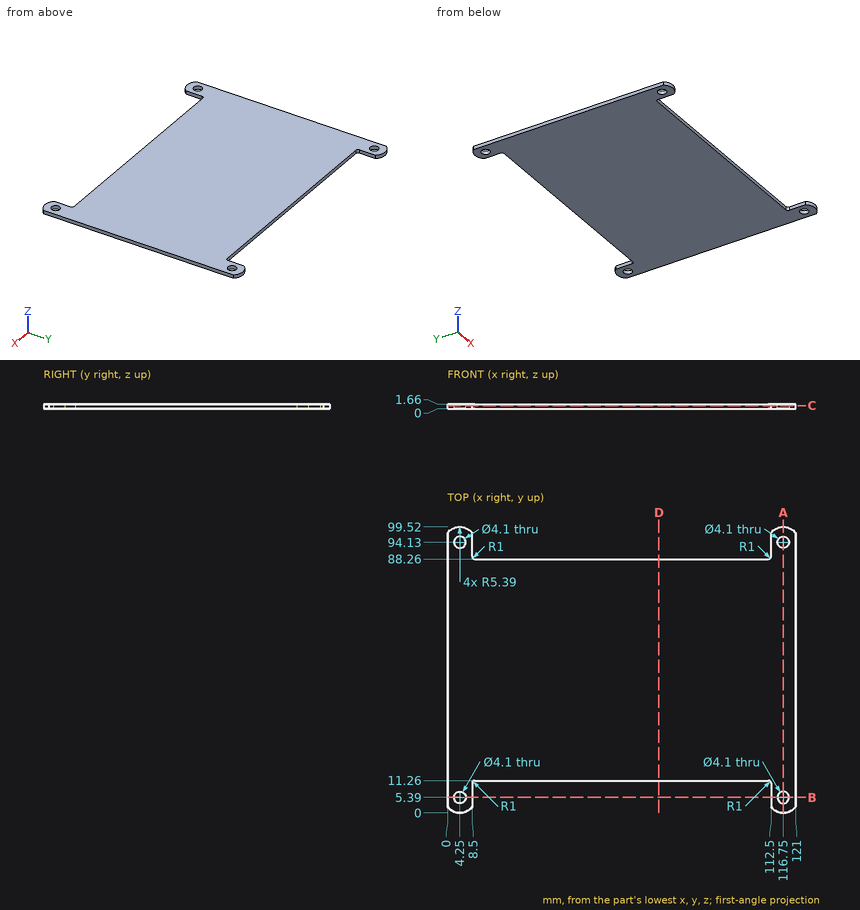
Verification items for this drawing (mm, ordinates from the low corner). Coordinates: 2 decimals unless noted, no trailing zeros. Write each loop counter-clockwise with the first axis right and the second up, starting at its lowest first coordinate (ties: lowest second). Pieces come first, ordered by that corner, then holes. Notation, with made-up numbers: (-18, 20.5) -> (8, 20.5) arc R26 cw to (8, 51.5) -> close; hole circle Ø11 at (78.5, 24.5). An arc over 180 degrees is marked (long way). One line per item, written item: value. Start each with the question number.
Q1. Cross-section at C-C on z = 1.1. Enter the section's corners in (x, y).
Q2. Thickness scan on L1, parallel to X at y = 94.13, z = 0.6; L2, parallel to X at y = 93.5, z = 0.35; L3, parallel to Y at x = 34.5, z = 0.4. Record the ranges inside material, lowest first. Write a range as from..to.
Q3. Cross-section at D-D on x = 73.5. Enter the section's corners in (y, z).
Q4. Cross-section at A-A on x = 116.75. Enter the section's corners in (y, z).
Q5. Cross-section at B-B on y = 5.39. Enter the section's corners in (x, z), and give its area (3 significant figures).
Checked values:
1. outline: (0, 2.07) arc R5.39 ccw to (8.5, 2.07) -> (8.5, 10.26) arc R1 cw to (9.5, 11.26) -> (111.5, 11.26) arc R1 cw to (112.5, 10.26) -> (112.5, 2.07) arc R5.39 ccw to (121, 2.07) -> (121, 97.45) arc R5.39 ccw to (112.5, 97.45) -> (112.5, 89.26) arc R1 cw to (111.5, 88.26) -> (9.5, 88.26) arc R1 cw to (8.5, 89.26) -> (8.5, 97.45) arc R5.39 ccw to (0, 97.45) -> close; hole circle Ø4.1 at (4.25, 5.39); hole circle Ø4.1 at (4.25, 94.13); hole circle Ø4.1 at (116.75, 5.39); hole circle Ø4.1 at (116.75, 94.13)
2. L1: x = 0..2.2, 6.3..8.5, 112.5..114.7, 118.8..121
2. L2: x = 0..2.3, 6.2..8.5, 112.5..114.8, 118.7..121
2. L3: y = 11.26..88.26
3. outline: (11.26, 0) -> (88.26, 0) -> (88.26, 1.66) -> (11.26, 1.66) -> close
4. outline: (0, 0) -> (3.34, 0) -> (3.34, 1.66) -> (0, 1.66) -> close; (7.44, 0) -> (92.08, 0) -> (92.08, 1.66) -> (7.44, 1.66) -> close; (96.18, 0) -> (99.52, 0) -> (99.52, 1.66) -> (96.18, 1.66) -> close
5. outline: (0, 0) -> (2.2, 0) -> (2.2, 1.66) -> (0, 1.66) -> close; (6.3, 0) -> (8.5, 0) -> (8.5, 1.66) -> (6.3, 1.66) -> close; (112.5, 0) -> (114.7, 0) -> (114.7, 1.66) -> (112.5, 1.66) -> close; (118.8, 0) -> (121, 0) -> (121, 1.66) -> (118.8, 1.66) -> close
5. area: 14.6 mm²
